from build123d import *

# Parameters (mm, degrees)
EXTRUDE1_DEPTH = 47.07
EXTRUDE2_DEPTH = 100
FILLET1_R      = 1


with BuildPart() as part:
    # Sketch1 → Revolve1 (revolve)
    with BuildSketch(Plane(origin=(0, 0, 0), x_dir=(0, 0, -1), z_dir=(1, 0, 0))):
        Polygon((0, 0), (-42.5, 0), (-42.5, 6.5), (-44.5, 6.5), (-44.5, 205.8), (-42.5, 205.8), (-42.5, 199.3), (0, 199.3), align=None)
    revolve(axis=Axis((0, 199.3, 0), (0, -1, 0)))

    # Sketch2 → Extrude1 (add)
    with BuildSketch(Plane.XZ.offset(-28.5)):
        with BuildLine():
            ThreePointArc((0, -17.430935144), (55.75, 0), (0, 17.430935144))
            ThreePointArc((0, 17.430935144), (-55.75, 0), (0, -17.430935144))
        make_face()
    extrude(amount=-EXTRUDE1_DEPTH)

    # Sketch3 → Extrude2 (add)
    with BuildSketch(Plane(origin=(0, 75.57, 0), x_dir=(-1, 0, 0), z_dir=(0, 1, 0))):
        with BuildLine():
            Line((48.03, 5), (48.03, -5))
            ThreePointArc((48.03, -5), (46.51379262, -6.562299411), (44.906801727, -5.093543292))
            ThreePointArc((44.906801727, -5.093543292), (44.566947891, -4.764619749), (44.209712274, -5.074577876))
            ThreePointArc((44.209712274, -5.074577876), (44.5, 0), (44.209712274, 5.074577876))
            ThreePointArc((44.209712274, 5.074577876), (44.566947891, 4.764619749), (44.906801727, 5.093543292))
            ThreePointArc((44.906801727, 5.093543292), (46.51379262, 6.562299411), (48.03, 5))
        make_face()
    extrude(amount=EXTRUDE2_DEPTH)

    # Fillet1
    fillet1_edges = [part.edges().sort_by_distance(p)[0] for p in [
        (-55.75, 28.5, 0),
        (-55.75, 75.57, 0),
        (55.75, 75.57, 0),
        (55.75, 28.5, 0),
    ]]
    fillet(fillet1_edges, radius=FILLET1_R)


solid = part.part
Input: part model. Units: mm. Frame: model coordinates. A direction names the side the tool comes from. Coordinates: 2 decimals unless noted, no trailing zeros. Order: outer loops, then holes, each group sorted by start corner. A loop starts at its lowest first (then second) coordinate and runs counter-clockwise, first axis right, second up.
1. Cut plane A-A, the plane x = 0. Return loops of the section in (y, z), plus the area to 3 significant figures.
Checked values:
outline: (0, -42.5) - (6.5, -42.5) - (6.5, -44.5) - (205.8, -44.5) - (205.8, -42.5) - (199.3, -42.5) - (199.3, 42.5) - (205.8, 42.5) - (205.8, 44.5) - (6.5, 44.5) - (6.5, 42.5) - (0, 42.5) - close
area: 17,700 mm2
2. Ray query, line 1 along X through (y, z) = (204, 0); line 2 along Y through (x, z) = (-45.5, 9.5). Return the intervals inside material, ascending.
Checked values:
line 1: x = -44.5 to -42.5, 42.5 to 44.5
line 2: y = 28.5 to 75.57
3. Contact query for flat-ended pins moving along their axis: P1, Ø1, axis at x = -26, z = 16, coming from the +Y side; P2, Ø8, axis at x = -26.5, y = 65, coming from the -Z side; P3, Ø1.9, axis at x = -47, z = 2, coming from the +Y side. Output: stop coordinate, or through.
Checked values:
P1: stops at y = 199.3
P2: stops at z = -38.39
P3: stops at y = 175.57
4. Cut plane D-D, the plane x = -24.5. Return loops of the section in (y, z).
Checked values:
outline: (0, -34.73) - (6.5, -34.73) - (6.5, -37.15) - (205.8, -37.15) - (205.8, -34.73) - (199.3, -34.73) - (199.3, 34.73) - (205.8, 34.73) - (205.8, 37.15) - (6.5, 37.15) - (6.5, 34.73) - (0, 34.73) - close
5. Draft query along Z for faces 6 (the flat face through (-1, 199.3, -1)), 7 (the flat face through (-47, 28.5, 0)), 8 (the cylindrical face through (-55.745, 51.72, 0.557)). Return one class per face: +Z half, -Z half, draft (parallel to the pull), parting line (faces both ways), or undercut.
Checked values:
face 6: undercut
face 7: draft
face 8: parting line
6. Cut plane C-C, the plane y = 100.5. Return loops of the section in (x, z), plus the area to 3 significant figures.
Checked values:
outline: (-48.03, -5) arc R1.56 ccw to (-44.91, -5.09) arc R0.35 cw to (-44.21, -5.07) arc R44.5 ccw (long way) to (-44.21, 5.07) arc R0.35 cw to (-44.91, 5.09) arc R1.56 ccw to (-48.03, 5) - close
area: 6,260 mm2
7. Cut plane B-B, the plane z = 0. Return loops of the section in (x, y).
Checked values:
outline: (-55.75, 29.5) arc R1 ccw to (-54.75, 28.5) - (-44.5, 28.5) - (-44.5, 6.5) - (-42.5, 6.5) - (-42.5, 0) - (42.5, 0) - (42.5, 6.5) - (44.5, 6.5) - (44.5, 28.5) - (54.75, 28.5) arc R1 ccw to (55.75, 29.5) - (55.75, 74.57) arc R1 ccw to (54.75, 75.57) - (44.5, 75.57) - (44.5, 205.8) - (42.5, 205.8) - (42.5, 199.3) - (-42.5, 199.3) - (-42.5, 205.8) - (-44.5, 205.8) - (-44.5, 175.57) - (-48.03, 175.57) - (-48.03, 75.57) - (-54.75, 75.57) arc R1 ccw to (-55.75, 74.57) - close
8. Access query for faces 1 (the cylindrical face through (25.861, 3.296, -33.727)), 2 (the flat face through (47, 75.57, 0)), 3 (the flat face through (47, 28.5, 0)), 4 (the flat face through (-48.03, 125, 0)), 5 (the cylindrical face through (25.861, 202.504, -33.727)). Directions: +Z, -Z, +X, -X, +Y, -Y. A direction counts if a zero-diameter tool reaches every point of the face in a straight line with its end or side. Return the directions, or none.
Checked values:
face 1: -Y
face 2: +X, +Y
face 3: +X, -Y
face 4: +Z, -Z, -X, +Y
face 5: +Y
